```python
from build123d import *


with BuildPart() as part:
    # Sketch → Revolution (revolve)
    with BuildSketch(Plane.XY):
        with BuildLine():
            Line((-68, 22), (-68, 20))
            Line((-70, 20), (-68, 20))
            Line((-70, 20), (-70, 2))
            Line((-70, 2), (-68, 2))
            Line((-68, 2), (-68, 0))
            Line((-68, 0), (0, 0))
            Line((0, 0), (0, 22))
            Line((0, 22), (-15, 22))
            ThreePointArc((-25, 12), (-17.928932, 14.928932), (-15, 22))
            Line((-57.5, 8.5), (-25, 12))
            ThreePointArc((-57.5, 13.5), (-60, 11), (-57.5, 8.5))
            Line((-57.5, 22), (-57.5, 13.5))
            Line((-68, 22), (-57.5, 22))
        make_face()
    revolve(axis=Axis((0, 0, 0), (0, 1, 0)))


solid = part.part
```
For this review, take the finished solid that the model builds, in its own axes (mm). A direction names the side the tool comes from. Coordinates: 2 decimals unless noted, no trailing zeros. Order: outer loops, then holes, each group sorted by start corner. A loop starts at its lowest first (then second) coordinate and runs counter-clockwise, first axis right, second up. Notation, with made-up numbers: (76.25, 89.5) -> (82.25, 89.5) arc R9 ccw to (82.25, 97.5) -> close; hole circle Ø3 at (60.5, 87.5). An arc over 180 degrees is marked (long way). Use CSV: the item, a comma, the result in double quotes. Start each with the question number.
Item 1: We need section B-B, the plane z = 0. Give the boundary of the cut face in (x, y), then the cut area to 3 significant figures.
Item 2: We need section C-C, the plane y = 4. Give the boundary of the cut face in (x, z).
Item 3: Draft analysis for pull direction Z (two halves, no side actions). For faces 1 (the face through (-36.556, 20.986, 57.338)), 2 (the face through (5.76, 11.83, -25.95)), 3 (the face through (12.465, 17.69, -56.133)), 4 (the face through (0, 22, 0)), state which applies: pulls with the +Z half, pulls with the -Z half, needs draft (parallel to the pull), parting line crosses it, or undercut.
Item 4: For faces 5 (the face through (-36.556, 0.986, 57.338)), 6 (the face through (11, 20, 68)), 7 (the face through (56, 22, 15)), list the 3-axis set-ups (+Z, -Z, +X, -X, +Y, -Y) from which the entire face can be reached by the end or side of a thin tool; tool diameter is ignored.
Item 5: We need section A-A, the plane x = 0. Give the boundary of the cut face in (y, z).
Item 6: Wall thickness on probe 1 along Z at (x, y) = (0, 19.75); probe 2 along Z at (x, y) = (0, 19); probe 3 along X at (y, z) = (16, -8.5): over which ranges is each line inside the solid? List them lowest first.
Item 7: Insertion check: pin 1 (1.5 mm diameter, centred on x = -51.5, y = 7, fed in from +Z); pin 2 (2 mm diameter, centred on x = 17, z = -24, fed in from +Y); pin 3 (3 mm diameter, centred on y = 3, z = -13.5, fed in from -X); pin 4 (6 mm diameter, centred on x = -22, z = -52.5, fed in from +Y). Each pin has a flat end and moves straight along its axis. Give the tip position at first contact, or say it passes through.
Derived:
1,outline,"(-70, 2) -> (-68, 2) -> (-68, 0) -> (68, 0) -> (68, 2) -> (70, 2) -> (70, 20) -> (68, 20) -> (68, 22) -> (57.5, 22) -> (57.5, 13.5) arc R2.5 cw to (57.5, 8.5) -> (25, 12) arc R10 cw to (15, 22) -> (-15, 22) arc R10 cw to (-25, 12) -> (-57.5, 8.5) arc R2.5 cw to (-57.5, 13.5) -> (-57.5, 22) -> (-68, 22) -> (-68, 20) -> (-70, 20) -> close"
1,area,"2,120 mm^2"
2,outline,"circle Ø140 at (0, 0)"
3,face 1,"parting line crosses it"
3,face 2,"undercut"
3,face 3,"undercut"
3,face 4,"needs draft"
4,face 5,"-Y"
4,face 6,"+Y"
4,face 7,"+Z, -Z, +X, -X, +Y"
5,outline,"(0, -68) -> (2, -68) -> (2, -70) -> (20, -70) -> (20, -68) -> (22, -68) -> (22, -57.5) -> (13.5, -57.5) arc R2.5 cw to (8.5, -57.5) -> (12, -25) arc R10 cw to (22, -15) -> (22, 15) arc R10 cw to (12, 25) -> (8.5, 57.5) arc R2.5 cw to (13.5, 57.5) -> (22, 57.5) -> (22, 68) -> (20, 68) -> (20, 70) -> (2, 70) -> (2, 68) -> (0, 68) -> close"
6,probe 1,"z = -70 to -57.5, -15.26 to 15.26, 57.5 to 70"
6,probe 2,"z = -70 to -57.5, -15.46 to 15.46, 57.5 to 70"
6,probe 3,"x = -69.48 to -56.87, -14.72 to 14.72, 56.87 to 69.48"
7,pin 1,"stops at z = 48.21"
7,pin 2,"stops at y = 11.63"
7,pin 3,"stops at x = -68.96"
7,pin 4,"stops at y = 22"
